Could you check a few things on this model? Use its own coordinates, in mm. Face numbers are marked on the shaded views. Coordinates: 2 decimals unless noted, no trailing zeros. Loops run counter-clockwise (first coordinate to the right, second up) from the corner with the lowest first, then second, coordinate; pieces in that order, holes last. Notation, with made-up numbers: (3, 65) - (61, 65) arc R30 cw to (61, 98) - close; hole circle Ø8 at (53.5, 0). An arc over 180 degrees is marked (long way). One line per item, written item: value. Start each with the question number.
(1) I'm going to push flat-ended pins straight in: P1, Ø1, axis at x = 6, y = 6.5, coming from the +Z side; P2, Ø12.5, axis at x = 0, z = 0, coming from the -Y side; P3, Ø1.5, axis at x = -1.5, y = 9, coming from the -Z side; P4, Ø2, axis at x = 8, y = 9, coming from the +Z side. Where does each tip first touch, or does it pass through?
(2) If we mould it in two halves opening along X, with no side actions, what happens to the marked faces 1, 2 and 3? For each: pulls with the +X half, pulls with the -X half, needs draft (parallel to the pull), parting line crosses it, or undercut.
(3) If we section it at C-C on y = 13.5: Write out the boundary of the cut face in (x, z) (1 decimal), then the cut area to 3 significant figures.
(4) If we section it at B-B on z = 0: Write out the boundary of the cut face in (x, y), then the cut area to 3 significant figures.
(5) If we section it at A-A on y = 11.5: Write out the boundary of the cut face in (x, z) (1 decimal).
(6) If I drill on line 1 along Z through (x, y) = (0, 6); line 2 along X through (y, z) = (6.75, 0); line 3 along X through (y, z) = (1, 4.5), over which ranges is the centre line in solid material (lowest first)? Write a range as from..to.
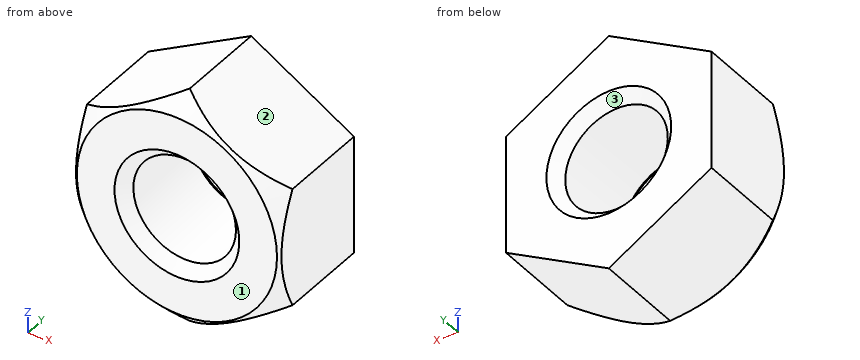
Solid Edge part; units mm, degrees
sketch "Sketch1" plane through (0, 0, 0) normal (0, -1, 0) x (1, 0, 0)
  circle A0 centre (0, 0) radius 16
extrude "Protrusion1" add sketch "Sketch1" against normal blind 14.4
chamfer "v_2" distance 2.5 angle 45 1 edges at (-16, 0, 0)
hole "Hole_1" at (0, 0, 0) direction (0, 1, 0) diameter 13.835 end up to next
chamfer "Chamfer_2" distance 1.5 angle 45 2 edges at (-6.9175, 0, 0) (0, 14.4, -6.9175)
sketch "Sketch2" plane through (0, 0, 0) normal (0, -1, 0) x (1, 0, 0)
  line L0 (0, 16) -> (-13.8564, 8)
extrude "ExtrudedCutout_1" cut sketch "Sketch2" against normal blind 70.3943 material side at (-6.9532, 0, 12.0433)
pattern_circular "Pattern1" count 6 over 360 about axis through (0, 0, 0) along (0, -1, 0) of "ExtrudedCutout_1"
Values:
1. P1: stops at z = 12.82
1. P2: passes through
1. P3: stops at z = -15.57
1. P4: stops at z = 11.96
2. face 1: needs draft
2. face 2: pulls with the +X half
2. face 3: undercut
3. outline: (-13.9, -8) - (0, -16) - (13.9, -8) - (13.9, 8) - (0, 16) - (-13.9, 8) - close; hole circle Ø15 at (0, 0)
3. area: 488 mm2
4. outline: (-13.86, 0.36) - (-13.5, 0) - (-8.42, 0) - (-6.92, 1.5) - (-6.92, 12.9) - (-8.42, 14.4) - (-13.86, 14.4) - close; (6.92, 1.5) - (8.42, 0) - (13.5, 0) - (13.86, 0.36) - (13.86, 14.4) - (8.42, 14.4) - (6.92, 12.9) - close
4. area: 195 mm2
5. outline: (-13.9, -8) - (0, -16) - (13.9, -8) - (13.9, 8) - (0, 16) - (-13.9, 8) - close; hole circle Ø13.8 at (0, 0)
6. line 1: z = -16..-6.92, 6.92..16
6. line 2: x = -13.86..-6.92, 6.92..13.86
6. line 3: x = -13.78..-5.9, 5.9..13.78
